from build123d import *

# Parameters (mm, degrees)
SKETCH1_W                 = 9.144
SKETCH1_H                 = 6.604
BOSS_EXTRUDE1_DEPTH       = 9.906
SKETCH4_W                 = 8.128
SKETCH4_H                 = 5.588
CUT_EXTRUDE1_DEPTH        = 8.382
CUT_EXTRUDE2_DEPTH        = 10.144
CUT_EXTRUDE4_REACH        = 8.604
SKETCH11_R                = 2.159
F_6_32_TAPPED_HOLE4_D     = 2.7051
F_6_32_TAPPED_HOLE4_DEPTH = 0.508


with BuildPart() as part:
    # Sketch1 → Boss-Extrude1 (new body)
    with BuildSketch(Plane.XY):
        with Locations((-3.267592039, 1.740807143)):
            Rectangle(SKETCH1_W, SKETCH1_H)
    extrude(amount=BOSS_EXTRUDE1_DEPTH)

    # Sketch4 → Cut-Extrude1 (cut)
    with BuildSketch(Plane.XY.offset(9.906)):
        with Locations((-3.267592039, 1.740807143)):
            Rectangle(SKETCH4_W, SKETCH4_H)
    extrude(amount=-CUT_EXTRUDE1_DEPTH, mode=Mode.SUBTRACT)

    # Sketch8 → Cut-Extrude2 (cut, through all)
    with BuildSketch(Plane.ZY.offset(7.839592039)):
        with BuildLine():
            Line((0, 5.042807143), (0, -1.561192857))
            ThreePointArc((0, -1.561192857), (0.381572084, 1.740807143), (0, 5.042807143))
        make_face()
    extrude(amount=-CUT_EXTRUDE2_DEPTH, mode=Mode.SUBTRACT)

    # Sketch11 → Cut-Extrude4 (cut, up to next)
    with BuildSketch(Plane(origin=(0, 5.042807143, 0), x_dir=(1, 0, 0), z_dir=(0, 1, 0)), mode=Mode.PRIVATE) as cut_extrude4_sk1:
        with Locations((-3.267592039, -6.985)):
            Circle(SKETCH11_R)
    cut_extrude4_tool1 = extrude(cut_extrude4_sk1.sketch, amount=-CUT_EXTRUDE4_REACH, mode=Mode.PRIVATE) & part.part
    add(cut_extrude4_tool1.solids().sort_by_distance((-3.267592, 5.042807, 6.985))[0], mode=Mode.SUBTRACT)

    # #6-32 Tapped Hole4
    with Locations(Plane(origin=(0, -1.561192857, 0), x_dir=(-1, 0, 0), z_dir=(0, -1, 0))):
        with Locations((3.267592039, -6.985)):
            Hole(F_6_32_TAPPED_HOLE4_D / 2, depth=F_6_32_TAPPED_HOLE4_DEPTH)


solid = part.part
Geometry: final body of the model. Coordinates: model frame, mm. A direction names the side the tool comes from. Round coordinates to 2 decimals unless told otherwise and drop trailing zeros. Loops run counter-clockwise (first coordinate to the right, second up) from the corner with the lowest first, then second, coordinate; pieces in that order, holes last. Notation, with made-up numbers: M -40,36 L 6,36 A28 cw 6,57 Z; hole C 33.25,6 d9. An arc over 180 degrees is marked long. Put each result on its own line as item: value. Start each with the question number.
(1) Section query A-A (x = -0.5). Return loops of the section in (y, z), then the cut area to 3 significant figures.
(2) Draft query along Z for faces 3 (the face through (-3.33, 1.69, 0.38)), 4 (the face through (-4.86, 4.79, 5.53)), 5 (the face through (-4, 4.7, 9.906)). Return one class per face: +Z half, -Z half, draft (parallel to the pull), parting line (faces both ways), or undercut.
(3) Section query D-D (x = -3.5). Return loops of the section in (y, z), then the cut area to 3 significant figures.
(4) Section query C-C (z = 3.25). Return loops of the section in (x, y), then the cut area to 3 significant figures.
(5) Material intervals for line 1 along X through (y, z) = (4.5, 8.5); line 2 along Y through (x, z) = (-1.25, 2.5); line 3 along Z through (x, y) = (-2.5, 2), sorted ascending. Write a range as [from, to].
(6) Set-up query: faces 1 (the face through (-3, -1.053, 5)), 2 (the face through (-3, 5.043, 4)). Return all of +Z, -Z, +X, -X, +Y, -Y with unobstructed straight access to the full face (end or side cutting, diameter ignored); none if empty.
(7) Contact query for flat-ended pins moving along their axis: pin 1 Ø1.7 at (x, y) = (-4.5, 2) entering from +Z; pin 2 Ø2.5 at (x, z) = (-3, 7) entering from +Y; pin 3 Ø2 at (x, z) = (-3.27, 6.98) entering from -Y. Output: stop coordinate, or through.
(8) Section query B-B (z = 7.25). Return loops of the section in (x, y).
Findings below:
1. outline: M -1.56,0 A14.48 cw 5.04,0 L 5.04,9.91 L 4.53,9.91 L 4.53,1.52 L -1.05,1.52 L -1.05,9.91 L -1.56,9.91 Z
1. area: 16.9 mm2
2. face 3: -Z half
2. face 4: undercut
2. face 5: +Z half
3. outline: M -1.56,0 A14.48 cw 5.04,0 L 5.04,4.84 L 4.53,4.84 L 4.53,1.52 L -1.05,1.52 L -1.05,5.65 L -1.56,5.65 Z; M -1.56,8.32 L -1.05,8.32 L -1.05,9.91 L -1.56,9.91 Z; M 4.53,9.13 L 5.04,9.13 L 5.04,9.91 L 4.53,9.91 Z
3. area: 13.4 mm2
4. outline: M -7.84,-1.56 L 1.3,-1.56 L 1.3,5.04 L -7.84,5.04 Z; hole M -7.33,-1.05 L 0.8,-1.05 L 0.8,4.53 L -7.33,4.53 Z
4. area: 15.0 mm2
5. line 1: x = [-7.84, -7.33], [0.8, 1.3]
5. line 2: y = [-1.56, -1.05], [4.53, 5.04]
5. line 3: z = [0.38, 1.52]
6. face 1: +Z
6. face 2: +Z, -Z, +X, -X, +Y
7. pin 1: stops at z = 1.52
7. pin 2: stops at y = -1.05
7. pin 3: passes through
8. outline: M -7.84,-1.56 L -4.59,-1.56 L -4.59,-1.05 L -7.33,-1.05 L -7.33,4.53 L -5.41,4.53 L -5.41,5.04 L -7.84,5.04 Z; M -1.94,-1.56 L 1.3,-1.56 L 1.3,5.04 L -1.12,5.04 L -1.12,4.53 L 0.8,4.53 L 0.8,-1.05 L -1.94,-1.05 Z
